from build123d import *

# Parameters (mm, degrees)
F0_W     = 51.2
F0_H     = 19.1
F1_DEPTH = 7
F3_W     = 1
F3_H     = 19.1
F4_DEPTH = 1
F5_W     = 1
F5_H     = 19.1
F6_DEPTH = 1
F7_R     = 0.25
F8_DEPTH = 5


with BuildPart() as f1:
    # F0 (on Top) → F1 (new body)
    with BuildSketch(Plane.XY):
        with Locations((-15.157956, -22.626161)):
            Rectangle(F0_W, F0_H)
    extrude(amount=F1_DEPTH)

    # F3 (on face) → F4 (join)
    with BuildSketch(Plane.XY.offset(7)):
        with Locations((-40.257956, -22.626161)):
            Rectangle(F3_W, F3_H)
    extrude(amount=F4_DEPTH)

    # F5 (on face) → F6 (join)
    with BuildSketch(Plane.XY.offset(7)):
        with Locations((9.942044, -22.626161)):
            Rectangle(F5_W, F5_H)
    extrude(amount=F6_DEPTH)

    # F7 (on face) → F8 (join)
    with BuildSketch(Plane.XY.offset(7)):
        with Locations((-15.157956, -15.006161)):
            Circle(F7_R)
        with Locations((-15.157956, -30.246161)):
            Circle(F7_R)
        with Locations((-12.617956, -15.006161)):
            Circle(F7_R)
        with Locations((-10.077956, -15.006161)):
            Circle(F7_R)
        with Locations((-17.697956, -15.006161)):
            Circle(F7_R)
        with Locations((-20.237956, -15.006161)):
            Circle(F7_R)
        with Locations((-12.617956, -30.246161)):
            Circle(F7_R)
        with Locations((-10.077956, -30.246161)):
            Circle(F7_R)
        with Locations((-7.537956, -30.246161)):
            Circle(F7_R)
        with Locations((-17.697956, -30.246161)):
            Circle(F7_R)
        with Locations((-20.237956, -30.246161)):
            Circle(F7_R)
        with Locations((-22.777956, -30.246161)):
            Circle(F7_R)
    extrude(amount=F8_DEPTH)


solid = f1.part
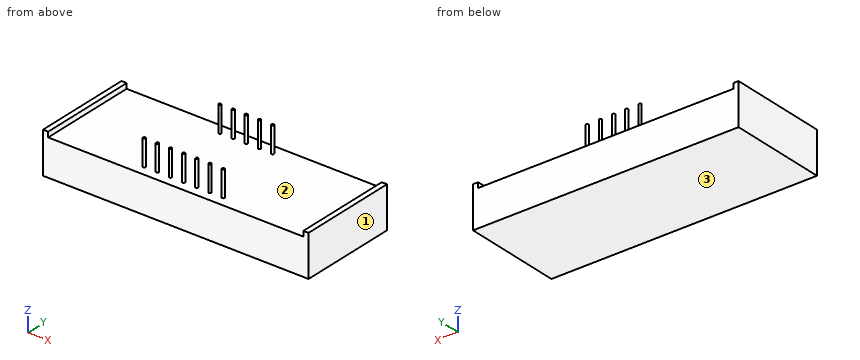
Can you work these out from the model? Positions are in its coordinate system, mm. Face numbers are marked on the shaded views. Give positions to 0.01 mm unless a question says otherwise; leave off trailing zeros. Loops run counter-clockwise (first coordinate to the right, second up) from the corner with the lowest first, then second, coordinate; pieces in that order, holes last. Notation, with made-up numbers: M 0.5,-6 L 57.5,-6 A17 cw 57.5,9 Z; hole C 58.5,73.5 d2. An arc over 180 degrees is marked long. One line per item, written item: value. Start each with the question number.
1) If we section it at B-B, the plane z = 11: Give the number of separate pieces and of enclosed holes in the cut face, and give its area (3 significant figures).
2) If we section it at A-A, the plane y = -27.5: Write out the boundary of the cut face in (x, z).
3) Thinking about a two-plate mould opening in X: for the marked faces 1, 2 and 3, which applies, +X half, -X half, draft (parallel to the pull), parting line (faces both ways), or undercut?
4) If I drill on line 1 (X direction, y = -24.75, z = 7.5); line 2 (Z direction, x = -19, y = -31), over which ranges is the centre line in solid material (lowest first)? Write a range as [from, to].
5) If we section it at C-C, the plane x = -19.5: Write out the boundary of the cut face in (y, z).
6) I'm going to push flat-ended pins straight in: pin 1 (5 mm diameter, centred on x = -27, z = 7.5, fed in from +Y); pin 2 (0.5 mm diameter, centred on x = -40, y = -19, fed in from +Z). Where does each tip first touch, or does it pass through?
Completed:
1. separate pieces: 12
1. enclosed holes: 0
1. area: 2.36 mm^2
2. outline: M -40.76,0 L 10.44,0 L 10.44,8 L 9.44,8 L 9.44,7 L -39.76,7 L -39.76,8 L -40.76,8 Z
3. face 1: +X half
3. face 2: undercut
3. face 3: draft
4. line 1: x = [-40.76, -39.76], [9.44, 10.44]
4. line 2: z = [0, 7]
5. outline: M -32.18,0 L -13.08,0 L -13.08,7 L -32.18,7 Z
6. pin 1: stops at y = -13.08
6. pin 2: stops at z = 8
